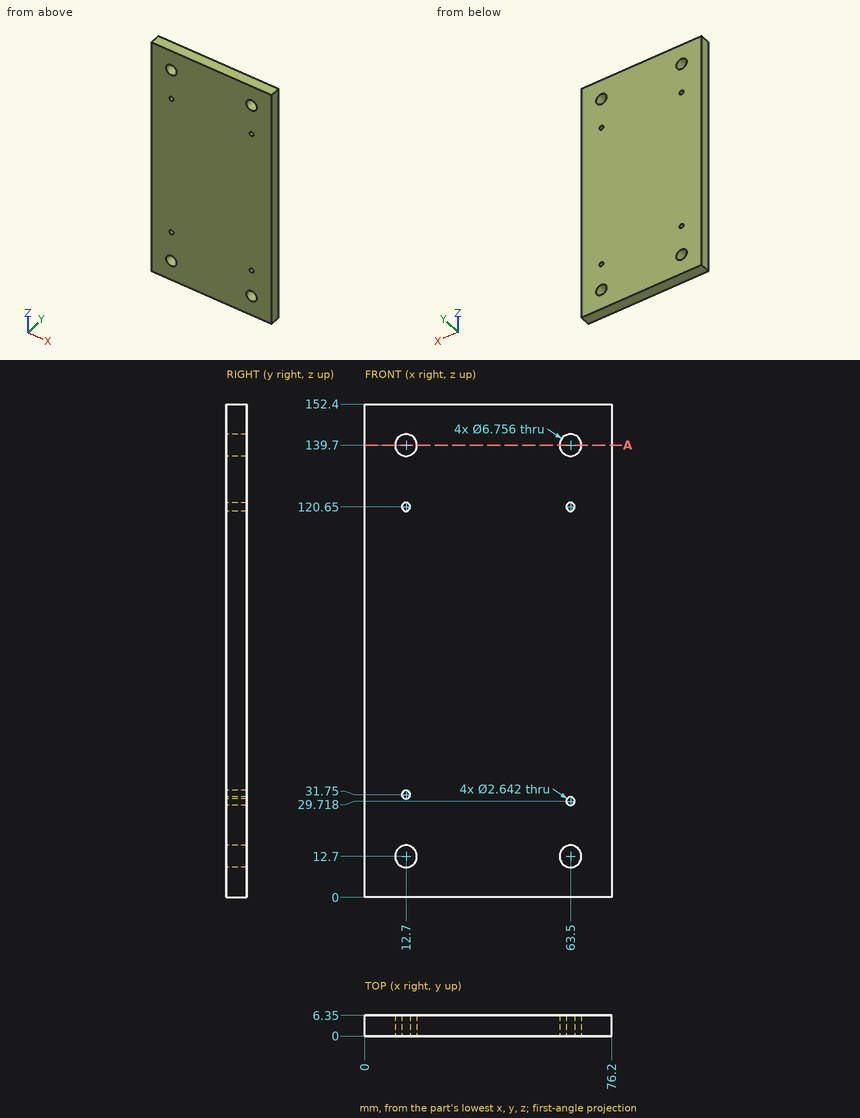
Could you check a few things on this drawing? It's one solid part, dimensions in mm from its lowest x, y, z. Give positions to 0.01 mm unless a question says otherwise; leave off trailing zeros. Write each loop counter-clockwise with the first axis right and the second up, starting at its lowest first coordinate (ties: lowest second). Pieces come first, ordered by that corner, then holes. Notation, with made-up numbers: (27.5, 15.5) -> (80.5, 15.5) arc R27 ccw to (80.5, 40.5) -> close; hole circle Ø11 at (-26, 70.25). An arc over 180 degrees is marked (long way). Write item = value, one per line.
(1) I need wall thicknesses on probe 1 along X at (y, z) = (3, 139.7); probe 2 along Z at (x, y) = (63.5, 4.5); probe 3 along X at (y, z) = (2, 120.65). Which ranges of each line are inside material? Lowest first, please. Write a range as from..to.
Worked out:
probe_1 = 0..9.32, 16.08..60.12, 66.88..76.2
probe_2 = 0..9.32, 16.08..28.4, 31.04..119.33, 121.97..136.32, 143.08..152.4
probe_3 = 0..11.38, 14.02..62.18, 64.82..76.2
(2) Suppose I cut it at A-A on z = 139.7. Write out the boundary of the cut face in (x, y).
Worked out:
outline = (0, 0) -> (9.32, 0) -> (9.32, 6.35) -> (0, 6.35) -> close; (16.08, 0) -> (60.12, 0) -> (60.12, 6.35) -> (16.08, 6.35) -> close; (66.88, 0) -> (76.2, 0) -> (76.2, 6.35) -> (66.88, 6.35) -> close
(3) I'm going to push a flat-ended pin straight in: P1, Ø1.6, axis at x = 63.5, z = 29.718, coming from the -Y side. Where does the tip first touch, or does it pass through?
Worked out:
P1 = through
